Verification items for the finished model (mm, model axes). Face numbers are marked on the shaded views. A direction names the side the tool comes from. Round coordinates to 2 decimals unless told otherwise and drop trailing zeros. Order: outer loops, then holes, each group sorted by start corner. A loop starts at its lowest first (then second) coordinate and runs counter-clockwise, first axis right, second up. Notation, with made-up numbers: (21, 42.5) -> (55, 42.5) arc R10 ccw to (55, 50.5) -> close; hole circle Ø4 at (58.5, 38). An arc over 180 degrees is marked (long way). Put each result on its own line as item: value.
from build123d import *

# Parameters (mm, degrees)
SKETCH1_W           = 520.7
SKETCH1_H           = 115
BOSS_EXTRUDE1_DEPTH = 9
BOSS_EXTRUDE2_DEPTH = 10
CUT_EXTRUDE1_DEPTH  = 9
CUT_EXTRUDE2_DEPTH  = 6
CUT_EXTRUDE3_DEPTH  = 2.5


with BuildPart() as part:
    # Sketch1 → Boss-Extrude1 (new body)
    with BuildSketch(Plane.XY):
        with Locations((0, 42.5)):
            Rectangle(SKETCH1_W, SKETCH1_H)
    extrude(amount=BOSS_EXTRUDE1_DEPTH)

    # Sketch2 → Boss-Extrude2 (add)
    with BuildSketch(Plane(origin=(0, 100, 0), x_dir=(1, 0, 0), z_dir=(0, 1, 0))):
        Polygon((-250.35, 10), (250.35, 10), (260.35, 0), (260.35, -9), (-260.35, -9), (-260.35, 0), align=None)
    extrude(amount=-BOSS_EXTRUDE2_DEPTH)

    # Sketch3 → Cut-Extrude1 (cut)
    with BuildSketch(Plane.XY.offset(9)):
        with BuildLine():
            Line((238.35, 88), (62.991811867, 88))
            ThreePointArc((62.991811867, 88), (55.920744055, 85.071067812), (52.991811867, 78))
            Line((52.991811867, 78), (52.991811867, 7))
            ThreePointArc((52.991811867, 7), (55.920744055, -0.071067812), (62.991811867, -3))
            Line((62.991811867, -3), (238.35, -3))
            ThreePointArc((238.35, -3), (245.421067812, -0.071067812), (248.35, 7))
            Line((248.35, 7), (248.35, 78))
            ThreePointArc((248.35, 78), (245.421067812, 85.071067812), (238.35, 88))
        make_face()
    cut_extrude1 = extrude(amount=-CUT_EXTRUDE1_DEPTH, mode=Mode.SUBTRACT)

    # Sketch4 → Cut-Extrude2 (cut)
    with BuildSketch(Plane.XY.offset(9)):
        with BuildLine():
            Line((62.991811867, -11), (238.35, -11))
            ThreePointArc((238.35, -11), (251.077922061, -5.727922061), (256.35, 7))
            Line((256.35, 7), (256.35, 78))
            ThreePointArc((256.35, 78), (251.077922061, 90.727922061), (238.35, 96))
            Line((238.35, 96), (62.991811867, 96))
            ThreePointArc((62.991811867, 96), (50.263889805, 90.727922061), (44.991811867, 78))
            Line((44.991811867, 78), (44.991811867, 7))
            ThreePointArc((44.991811867, 7), (50.263889805, -5.727922061), (62.991811867, -11))
        make_face()
    cut_extrude2 = extrude(amount=-CUT_EXTRUDE2_DEPTH, mode=Mode.SUBTRACT)

    # Mirror1: Cut-Extrude1, Cut-Extrude2 across plane
    add(cut_extrude1.mirror(Plane(origin=(0, 0, 0), x_dir=(0, 0, 1), z_dir=(1, 0, 0))), mode=Mode.SUBTRACT)
    add(cut_extrude2.mirror(Plane(origin=(0, 0, 0), x_dir=(0, 0, 1), z_dir=(1, 0, 0))), mode=Mode.SUBTRACT)

    # Sketch5 → Cut-Extrude3 (cut)
    with BuildSketch(Plane(origin=(0, 100, 0), x_dir=(1, 0, 0), z_dir=(0, 1, 0))):
        with BuildLine():
            Line((-250.35, 5), (250.35, 5))
            ThreePointArc((250.35, 5), (252.263417162, 5.380602337), (253.885533906, 6.464466094))
            Line((253.885533906, 6.464466094), (260.249494937, 0.100505063))
            ThreePointArc((260.249494937, 0.100505063), (255.707568053, -2.934313455), (250.35, -4))
            Line((250.35, -4), (-250.35, -4))
            ThreePointArc((-250.35, -4), (-255.707568053, -2.934313455), (-260.249494937, 0.100505063))
            Line((-260.249494937, 0.100505063), (-253.885533906, 6.464466094))
            ThreePointArc((-253.885533906, 6.464466094), (-252.263417162, 5.380602337), (-250.35, 5))
        make_face()
    extrude(amount=-CUT_EXTRUDE3_DEPTH, mode=Mode.SUBTRACT)


solid = part.part
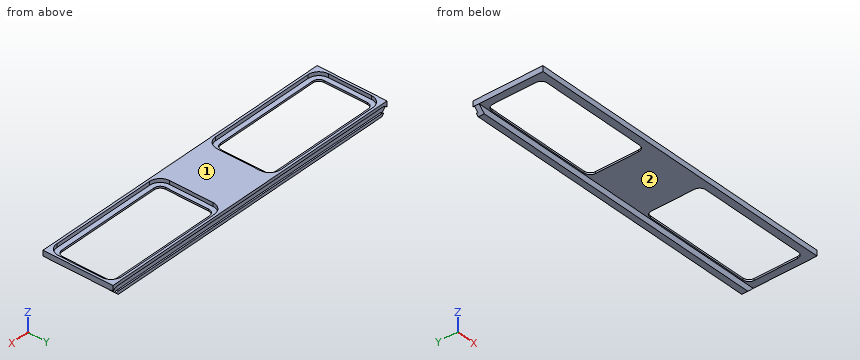
Item 1: Section check A-A on x = 183.5. Record the boundary of the cut face in (y, z), then the cut area to 4 significant figures.
Check sheet entries:
outline: (-15, 0) -> (-3, 0) -> (-3, 3) -> (-11, 3) -> (-11, 9) -> (-15, 9) -> close; (88, 0) -> (90, 0) -> (90, -10) -> (100, -10) -> (100, -5) -> (97.5, -5) -> (97.5, 4) -> (100, 4) -> (100, 9) -> (96, 9) -> (96, 3) -> (88, 3) -> close
area: 197.5 mm^2
Item 2: Gauge pin test, flat end, axial feed: pin 1 Ø3 at (x, z) = (-1.5, 0) entering from +Y. Record the tip position at first contact, or that the pin passes through.
Check sheet entries:
pin 1: stops at y = 97.5
Item 3: Section check B-B on y = 17.5. Record the boundary of the cut face in (x, z).
Check sheet entries:
outline: (-260.35, 0) -> (-248.35, 0) -> (-248.35, 3) -> (-256.35, 3) -> (-256.35, 9) -> (-260.35, 9) -> close; (-52.99, 0) -> (52.99, 0) -> (52.99, 3) -> (44.99, 3) -> (44.99, 9) -> (-44.99, 9) -> (-44.99, 3) -> (-52.99, 3) -> close; (248.35, 0) -> (260.35, 0) -> (260.35, 9) -> (256.35, 9) -> (256.35, 3) -> (248.35, 3) -> close
Item 4: Tool access check on the marked faces 1 and 2. Record the directions out of +Z, -Z, +X, -X, +Y, -Y that give a thin tool (end or side, any length) a straight path to the whole face; none if there is none.
Check sheet entries:
face 1: +Z, +X, -X, +Y, -Y
face 2: -Z, +X, -X, -Y
Item 5: Material ranges on L1, parallel to X at y = 77.5, z = 1; L2, parallel to X at y = 64.5, z = 5.25; L3, parallel to Y at x = 189.5, z = 3.5, recorded low to high. Write a range as [from, to].
Check sheet entries:
L1: x = [-260.35, -248.35], [-52.99, 52.99], [248.35, 260.35]
L2: x = [-260.35, -256.35], [-44.99, 44.99], [256.35, 260.35]
L3: y = [-15, -11], [96, 97.5]
